from build123d import *

# Parameters (mm, degrees)
F0_R     = 6.35
F1_DEPTH = 19.05


with BuildPart() as f1:
    # F0 (on Top) → F1 (new body)
    with BuildSketch(Plane.XY):
        with BuildLine():
            ThreePointArc((0.332687, -44.448755), (31.5483, -31.313053), (44.45, 0))
            ThreePointArc((44.45, 0), (30.100022, 32.707663), (-3.684587, 44.297024))
            ThreePointArc((-3.684587, 44.297024), (-44.404528, -2.010069), (0.332687, -44.448755))
        make_face()
        Circle(F0_R, mode=Mode.SUBTRACT)
        with BuildLine():
            ThreePointArc((678.049984, 261.737104), (619.235303, 345.391653), (520.612783, 318.357437))
            ThreePointArc((520.612783, 318.357437), (526.551405, 198.613195), (646.341094, 193.675463))
            ThreePointArc((646.341094, 193.675463), (669.73379, 224.194326), (678.049984, 261.737104))
        make_face()
        with BuildLine():
            ThreePointArc((-3.684587, 44.297024), (30.100022, 32.707663), (44.45, 0))
            ThreePointArc((44.45, 0), (31.5483, -31.313053), (0.332687, -44.448755))
            ThreePointArc((0.332687, -44.448755), (344.122424, 18.224174), (646.341094, 193.675463))
            ThreePointArc((646.341094, 193.675463), (526.551405, 198.613195), (520.612783, 318.357437))
            ThreePointArc((520.612783, 318.357437), (286.146598, 128.368607), (-3.684587, 44.297024))
        make_face()
    extrude(amount=F1_DEPTH)


solid = f1.part
Could you check a few things on this model? Use its own coordinates, in mm. Coordinates: 2 decimals unless noted, no trailing zeros. Loops run counter-clockwise (first coordinate to the right, second up) from the corner with the lowest first, then second, coordinate; pieces in that order, holes last.
1. For P1, Ø10, axis at y = 161, z = 4, coming from the -X side; P2, Ø8, axis at x = 477.5, z = 3.5, coming from the -Y side; P3, Ø10, axis at x = 0, y = 0, coming from the +Z side; P4, Ø3, axis at y = 23, z = 2, coming from the -X side, each with a flat end and sliding along its axis, tell me the tip position at first contact or that it passes through.
2. I need wall thicknesses on L1, parallel to Y at x = 0, z = 11.25; L2, parallel to Y at x = 226, z = 8.75 (3 decimals); L3, parallel to Y at x = 648.5, z = 9.25. Which ranges of each line are inside material? Lowest first, please.
3. Imagine slicing it at C-C (y = 155.5). Please give me the cut outline in (x, z), and give its area (3 significant figures).
4. We'd pull the mould along Y, two halves only. Please class faces 1 (the face through (369, 139, 19.05)), 2 (the face through (-1.38, -6.2, 9.39)), 3 (the face through (-44.437, -1.057, 9.392)): released by +Y, released by -Y, zero draft, split by the parting line, or undercut.
5. Imagine slicing it at A-A (z = 15.25). Please give me the cut outline in (x, y), and give its area (3 significant figures).
6. Imagine slicing it at B-B (x = 252). Please give me the cut outline in (y, z), and give its area (3 significant figures).
Computed values:
1. P1: stops at x = 334.6
1. P2: stops at y = 76.47
1. P3: passes through
1. P4: stops at x = -38.9
2. L1: y = -44.45 to -6.35, 6.35 to 44.61
2. L2: y = -17.335 to 100.195
2. L3: y = 195.55 to 327.92
3. outline: (333.79, 0) - (598.01, 0) - (598.01, 19.05) - (333.79, 19.05) - close
3. area: 5,030 mm2
4. face 1: zero draft
4. face 2: undercut
4. face 3: split by the parting line
5. outline: (-3.68, 44.3) arc R44.45 ccw to (0.33, -44.45) arc R1016 ccw to (646.34, 193.68) arc R88.9 ccw to (678.05, 261.74) arc R88.9 ccw to (520.61, 318.36) arc R762 cw to start; hole circle Ø12.7 at (0, 0)
5. area: 99,700 mm2
6. outline: (-10.84, 0) - (111.59, 0) - (111.59, 19.05) - (-10.84, 19.05) - close
6. area: 2,330 mm2
